Could you check a few things on this model? Use its own coordinates, in mm. Face numbers are marked on the shaded views. A direction names the side the tool comes from. Coordinates: 2 decimals unless noted, no trailing zeros. Loops run counter-clockwise (first coordinate to the right, second up) from the corner with the lowest first, then second, coordinate; pieces in that order, holes last. Notation, with made-up numbers: M 14,49.25 L 28,49.25 A24 cw 28,65.25 Z; hole C -9,25 d7. An arc over 180 degrees is marked long. Return JSON: item names as keys, results as strings. Group by question number.
from build123d import *

# Parameters (mm, degrees)
F1_DEPTH  = 20
F2_R      = 10
F3_R      = 20
F5_D      = 8.8
F6_W      = 10
F6_H      = 40
F7_DEPTH  = 12
F8_R      = 9
F9_DEPTH  = 17
F11_D     = 3.3
F11_DEPTH = 10
F11_TIP   = 0.9914200214


with BuildPart() as f1:
    # F0 (on Front) → F1 (new body)
    with BuildSketch(Plane.XZ):
        Polygon((39.4714460536, 44.5363200395), (-40.3757039464, 44.5363200395), (-40.3757039464, 4.5363200395), (9.6242960536, 4.5363200395), (9.6242960536, -56.8236818447), (39.4714460536, -56.8236818447), align=None)
    extrude(amount=F1_DEPTH)

    # F2
    f2_edges = [f1.edges().sort_by_distance(p)[0] for p in [
        (9.624296, -10, 4.53632),
    ]]
    fillet(f2_edges, radius=F2_R)

    # F3
    f3_edges = [f1.edges().sort_by_distance(p)[0] for p in [
        (39.471446, -10, 44.53632),
    ]]
    fillet(f3_edges, radius=F3_R)

    # F5 (through all)
    with Locations(Plane.YZ.offset(39.4714460536)):
        with Locations((-10, -46.8236818447)):
            Hole(F5_D / 2)

    # F6 (on face) → F7 (cut)
    with BuildSketch(Plane(origin=(-40.3757039464, 0, 0), x_dir=(0, -1, 0), z_dir=(-1, 0, 0))):
        with Locations((10, 24.5363200395)):
            Rectangle(F6_W, F6_H)
    extrude(amount=-F7_DEPTH, mode=Mode.SUBTRACT)

    # F8 (on face) → F9 (cut)
    with BuildSketch(Plane.XZ.offset(20)):
        with Locations((-23.3757039464, 24.5363200395)):
            Circle(F8_R)
    extrude(amount=-F9_DEPTH, mode=Mode.SUBTRACT)

    # F11
    with Locations(Plane(origin=(-40.3757039464, 0, 0), x_dir=(0, -1, 0), z_dir=(-1, 0, 0))):
        with Locations((2.5, 39.5363200395), (17.5, 39.5363200395), (17.5, 9.5363200395), (2.5, 9.5363200395)):
            Hole(F11_D / 2, depth=F11_DEPTH)
            with Locations((0, 0, -(F11_DEPTH + F11_TIP / 2))):  # 118° drill point
                Cone(0, F11_D / 2, F11_TIP, mode=Mode.SUBTRACT)


solid = f1.part
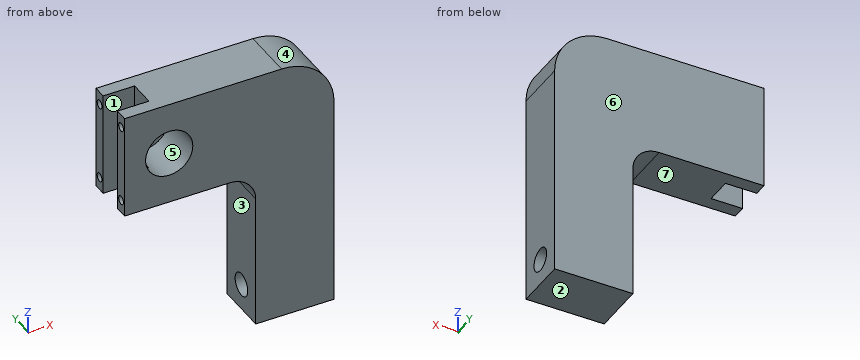
(1) Will these pins go through, and if not, where does the flat tip stop? P1, Ø12, axis at x = -19.5, z = 17, coming from the -Y side; P2, Ø5, axis at x = -24, y = -6.5, coming from the -Z side; P3, Ø3, axis at y = -17.5, z = 39.54, coming from the -X side; P4, Ø8, axis at y = -8, z = -7.5, coming from the -X side.
(2) If I drill on L1, parallel to Z at x = -34.25, y = -2.5; L2, parallel to Z at x = -23, y = -10.75; L3, parallel to X at y = -3.75, z = 17.5, over which ranges is the centre line in solid material (lowest first)? Write a range as [from, to].
(3) Imagine slicing it at C-C, the plane x = -18. Write out the boundary of the cut face in (y, z), then the cut area to 3 significant figures.
(4) Imagine slicing it at A-A, the plane y = -10. Write out the boundary of the cut face in (x, z).
(5) We'd pull the mould along Z, two halves only. Please class the marked faces 4, 5, 6 and 7: +Z half, -Z half, draft (parallel to the pull), parting line (faces both ways), or undercut.
(6) For the marked faces 1, 2 and 3, which set-ups out of +Z, -Z, +X, -X, +Y, -Y let a thin tool reach every point of the face, with its end or its side?
(7) Imagine slicing it at B-B, the plane x = 14. Write out the boundary of the cut face in (y, z).
(8) Imagine slicing it at D-D, the plane z = -39.5. Write out the boundary of the cut face in (x, y), then the cut area to 3 significant figures.
Checks:
{
 "1": {"P1": "y = -20", "P2": "z = 4.54", "P3": "x = -30.29", "P4": "x = 9.43"},
 "2": {"L1": "[4.54, 7.89], [11.19, 37.89], [41.19, 44.54]", "L2": "[4.54, 15.54], [33.53, 44.54]", "L3": "[-40.38, -28.99], [-17.76, 39.47]"},
 "3": {"outline": "M -20,4.54 L 0,4.54 L 0,44.54 L -20,44.54 L -20,31.75 L -3,31.75 L -3,17.32 L -20,17.32 Z", "area": "555 mm²"},
 "4": {"outline": "M -28.38,4.54 L -0.38,4.54 A10 cw 9.62,-5.46 L 9.62,-42.42 L 39.47,-42.42 L 39.47,24.54 A20 ccw 19.47,44.54 L -28.38,44.54 L -28.38,32.02 A9 cw long -28.38,17.05 Z; M 9.62,-56.82 L 39.47,-56.82 L 39.47,-51.22 L 9.62,-51.22 Z"},
 "5": {"face 4": "+Z half", "face 5": "undercut", "face 6": "draft", "face 7": "-Z half"},
 "6": {"face 1": "+Z, -Z, -X", "face 2": "-Z, +X, -X, +Y, -Y", "face 3": "-Z, -X, +Y, -Y"},
 "7": {"outline": "M -20,-56.82 L 0,-56.82 L 0,44.54 L -20,44.54 Z; hole C -10,-46.82 d8.8"},
 "8": {"outline": "M 9.62,-20 L 39.47,-20 L 39.47,0 L 9.62,0 Z", "area": "597 mm²"}
}
